Part model, mm, in its own coordinate system. A direction names the side the tool comes from. Round coordinates to 2 decimals unless told otherwise and drop trailing zeros. Write each loop counter-clockwise with the first axis right and the second up, starting at its lowest first coordinate (ties: lowest second). Pieces come first, ordered by that corner, then holes.
1) Pull direction Y, two halves, no side cores. Call faces 1 (the cylindrical face through (42.541, 13.606, 12.522)), 2 (the flat face through (0, 50, 13)), 3 (the cylindrical face through (110.992, 38.103, 12.979)): +Y half, -Y half, draft (parallel to the pull), parting line (faces both ways), or undercut.
2) Saw through at D-D on y = 41.5. Write the cut outline in (x, z).
3) Saw through at B-B on y = 64. Write the cut outline in (x, z).
4) Saw through at C-C on x = 40. Write the cut outline in (y, z).
5) Saw through at A-A on z = 12.7. Write the cut outline in (x, y), and give its area (3 significant figures).
6) Flat gauge pins, fed straight in: pin 1 (2 mm diameter, centred on x = 103, z = 17.5, fed in from -Y); pin 2 (7.5 mm diameter, centred on x = 20, z = 17, fed in from +Y); pin 3 (7.5 mm diameter, centred on y = 27, z = 7, fed in from +X). Where does each tip first touch, or does it go through?
7) Which spindle directions (+Z, -Z, +X, -X, +Y, -Y) get a long thin tool onto all of the face, cutting with end or side? Do faces 4 (the cylindrical face through (44.5, 111, 13.5)), 5 (the cylindrical face through (38.103, 110.992, 12.421)), 6 (the flat face through (101.6, 51, 13)). Say none if no direction does.
8) Drill centre lines: L1, parallel to Z at x = 50.8, y = 106.5; L2, parallel to Y at x = 50.8, z = 9; L3, parallel to X at y = 108, z = 12.7. Where is each one in solid material? Low to high.
```python
from build123d import *

# Parameters (mm, degrees)
SKETCH2_W           = 101.6
SKETCH2_H           = 101.6
SKETCH2_R           = 38.1
BOSS_EXTRUDE1_DEPTH = 25.4
SKETCH3_R           = 6.35
BOSS_EXTRUDE2_DEPTH = 19.05
SKETCH4_R           = 6.35
BOSS_EXTRUDE3_DEPTH = 19.05


with BuildPart() as part:
    # Sketch2 → Boss-Extrude1 (new body)
    with BuildSketch(Plane.XY):
        with Locations((50.8, 50.8)):
            Rectangle(SKETCH2_W, SKETCH2_H)
        with Locations((50.8, 50.8)):
            Circle(SKETCH2_R, mode=Mode.SUBTRACT)
    extrude(amount=BOSS_EXTRUDE1_DEPTH)

    # Sketch3 → Boss-Extrude2 (add)
    with BuildSketch(Plane(origin=(0, 101.6, 0), x_dir=(1, 0, 0), z_dir=(0, 1, 0))):
        with BuildLine():
            Line((101.6, -25.4), (101.6, 0))
            Line((101.6, 0), (50.8, 0))
            ThreePointArc((50.8, 0), (38.1, -12.7), (50.8, -25.4))
            Line((50.8, -25.4), (101.6, -25.4))
        make_face()
        with Locations(Location((50.8, -12.7, 0), (0, 0, 90))):
            Circle(SKETCH3_R, mode=Mode.SUBTRACT)
    extrude(amount=BOSS_EXTRUDE2_DEPTH)

    # Sketch4 → Boss-Extrude3 (add)
    with BuildSketch(Plane(origin=(101.6, 0, 0), x_dir=(0, 0, -1), z_dir=(1, 0, 0))):
        with BuildLine():
            Line((0, 120.65), (-25.4, 120.65))
            Line((-25.4, 120.65), (-25.4, 50.8))
            ThreePointArc((-25.4, 50.8), (-12.7, 38.1), (0, 50.8))
            Line((0, 50.8), (0, 120.65))
        make_face()
        with Locations(Location((-12.7, 50.8, 0), (0, 0, 180))):
            Circle(SKETCH4_R, mode=Mode.SUBTRACT)
    extrude(amount=BOSS_EXTRUDE3_DEPTH)


solid = part.part
```
Completed:
1. face 1: undercut
1. face 2: draft
1. face 3: -Y half
2. outline: (0, 0) - (13.85, 0) - (13.85, 25.4) - (0, 25.4) - close; (87.75, 0) - (101.6, 0) - (101.6, 4.05) - (120.65, 4.05) - (120.65, 21.35) - (101.6, 21.35) - (101.6, 25.4) - (87.75, 25.4) - close
3. outline: (0, 0) - (15.06, 0) - (15.06, 25.4) - (0, 25.4) - close; (86.54, 0) - (120.65, 0) - (120.65, 25.4) - (86.54, 25.4) - close
4. outline: (0, 0) - (14.26, 0) - (14.26, 25.4) - (0, 25.4) - close; (87.34, 0) - (101.6, 0) - (101.6, 6.02) - (120.65, 6.02) - (120.65, 19.38) - (101.6, 19.38) - (101.6, 25.4) - (87.34, 25.4) - close
5. outline: (0, 0) - (101.6, 0) - (101.6, 38.1) - (120.65, 38.1) - (120.65, 44.45) - (101.6, 44.45) - (101.6, 57.15) - (120.65, 57.15) - (120.65, 120.65) - (57.15, 120.65) - (57.15, 101.6) - (44.45, 101.6) - (44.45, 120.65) - (38.1, 120.65) - (38.1, 101.6) - (0, 101.6) - close; hole circle Ø76.2 at (50.8, 50.8)
5. area: 8,060 mm2
6. pin 1: stops at y = 38.68
6. pin 2: stops at y = 101.6
6. pin 3: stops at x = 101.6
7. face 4: +Y
7. face 5: -X, +Y
7. face 6: +X
8. L1: z = 0 to 6.35, 19.05 to 25.4
8. L2: y = 0 to 12.7, 88.9 to 101.6
8. L3: x = 38.1 to 44.45, 57.15 to 120.65
